```python
from build123d import *

# Parameters (mm, degrees)
F0_R     = 2.38125
F1_DEPTH = 17.4625


with BuildPart() as f1:
    # F0 (on Front) → F1 (new body)
    with BuildSketch(Plane.XZ):
        with BuildLine():
            Line((-304.8, 0), (0, 0))
            Line((0, 0), (-13.828941, 87.3125))
            Line((-13.828941, 87.3125), (-254, 87.3125))
            ThreePointArc((-254, 87.3125), (-289.921024, 72.433524), (-304.8, 36.5125))
            Line((-304.8, 36.5125), (-304.8, 0))
        make_face()
        with Locations((-273.05, 31.75)):
            Circle(F0_R, mode=Mode.SUBTRACT)
    extrude(amount=F1_DEPTH)


solid = f1.part
```
The listing builds one solid part. Answer for the finished solid, in the listing's coordinates (mm). Give positions to 0.01 mm unless a question says otherwise; leave off trailing zeros. Loops run counter-clockwise (first coordinate to the right, second up) from the corner with the lowest first, then second, coordinate; pieces in that order, holes last. Notation, with made-up numbers: (45, 28.5) - (84, 28.5) arc R12 ccw to (84, 40.5) - close; hole circle Ø11 at (9, 26.25). An arc over 180 degrees is marked (long way). Answer as CSV lines item,"result". Start each with the question number.
Item 1: A cutting plane is placed at C-C on z = 54.5. Determine the outline of the cut face in (x, y).
Item 2: A cutting plane is placed at A-A on y = -12.25. Determine the outline of the cut face in (x, z), then the cut area to 3 significant figures.
Item 3: Each of these flat-tipped pins is pushed along its axis until it touches: pin 1 (5 mm diameter, centred on y = -13, z = 68.5, fed in from -X); pin 2 (8 mm diameter, centred on y = -5.5, z = 41, fed in from +X); pin 3 (3 mm diameter, centred on x = -273.05, z = 31.75, fed in from -Y). Where does it stop, or does it pass through?
Item 4: A cutting plane is placed at B-B on z = 67. Determine the outline of the cut face in (x, y).
Item 5: Find the intervals of material crossed by line 1 (Z direction, x = -273.05, y = -9.5); line 2 (X direction, y = -6, z = 16); line 3 (X direction, y = -11.5, z = 7), in increasing order. Write a range as from..to.
Found:
1,outline,"(-301.51, -17.46) - (-8.63, -17.46) - (-8.63, 0) - (-301.51, 0) - close"
2,outline,"(-304.8, 0) - (0, 0) - (-13.83, 87.31) - (-254, 87.31) arc R50.8 ccw to (-304.8, 36.51) - close; hole circle Ø4.76 at (-273.05, 31.75)"
2,area,"25,400 mm^2"
3,pin 1,"stops at x = -295.37"
3,pin 2,"stops at x = -5.86"
3,pin 3,"passes through"
4,outline,"(-294.63, -17.46) - (-10.61, -17.46) - (-10.61, 0) - (-294.63, 0) - close"
5,line 1,"z = 0..29.37, 34.13..83.61"
5,line 2,"x = -304.8..-2.53"
5,line 3,"x = -304.8..-1.11"
